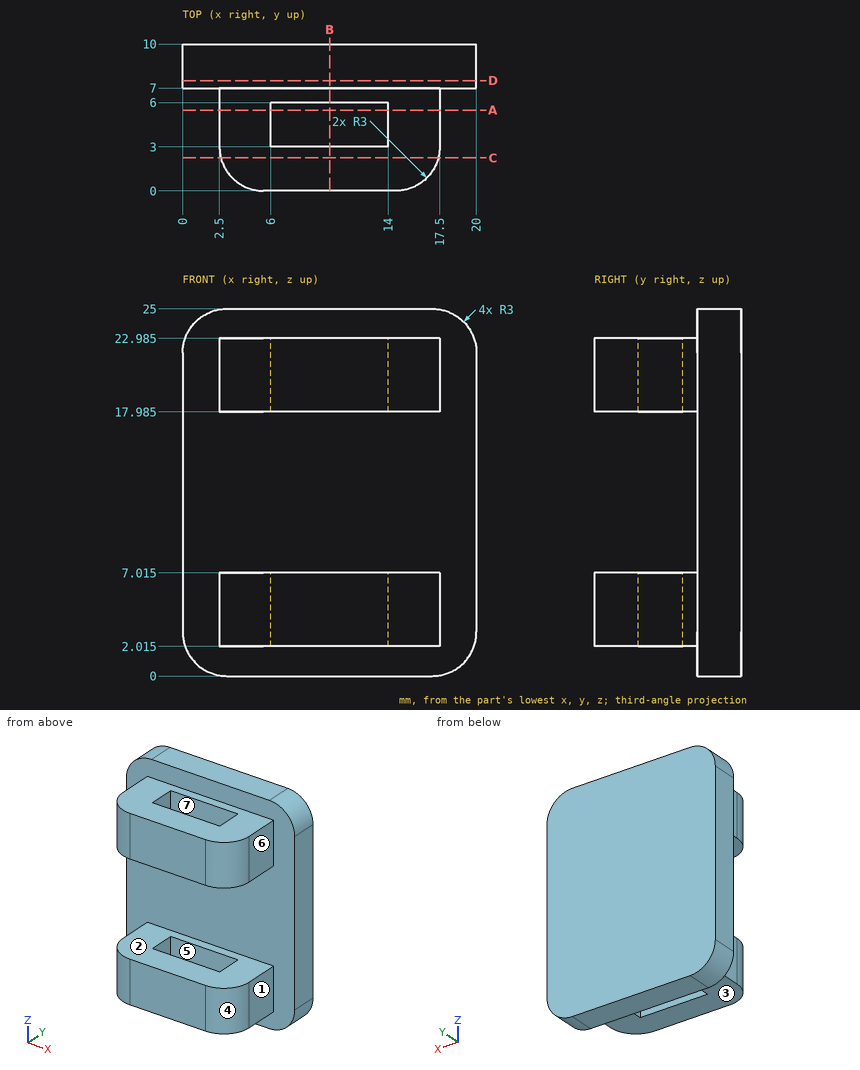
Part print with two shaded views. Sizes in mm from the minimum x, y, z corner. A direction names the side the tool comes from. Give positions to 0.01 mm unless a question says otherwise; leave off trailing zeros. Order: outer loops, then holes, each group sorted by start corner. A loop starts at its lowest first (then second) coordinate and runs counter-clockwise, first axis right, second up. Notation, with made-up numbers: M 67,76 L 125,76 A7 ccw 125,82 Z; hole C 39,3.25 d2. An arc over 180 degrees is marked long. Write item = value, one per line.
Q1. Cut at B-B, the plane x = 10. List the corners of the cut face in (y, z) (3 decimals).
Derived:
outline = M 0,2.015 L 3,2.015 L 3,7.015 L 0,7.015 Z; M 0,17.985 L 3,17.985 L 3,22.985 L 0,22.985 Z; M 6,2.015 L 7,2.015 L 7,0 L 10,0 L 10,25 L 7,25 L 7,22.985 L 6,22.985 L 6,17.985 L 7,17.985 L 7,7.015 L 6,7.015 Z
Q2. Drill centre lines: line 1 (Y direction, x = 11.25, z = 6); line 2 (Z direction, x = 16, y = 3) (3 decimals); line 3 (X direction, y = 5, z = 6). Where is each one in solid material? Low to high. Write a range as [from, to].
Derived:
line_1 = [0, 3], [6, 10]
line_2 = [2.015, 7.015], [17.985, 22.985]
line_3 = [2.5, 6], [14, 17.5]
Q3. Cut at C-C, the plane y = 2.25. List the corners of the cut face in (x, z) (3 decimals), then the cut area to 3 significant figures.
Derived:
outline = M 2.595,2.015 L 17.405,2.015 L 17.405,7.015 L 2.595,7.015 Z; M 2.595,17.985 L 17.405,17.985 L 17.405,22.985 L 2.595,22.985 Z
area = 148 mm2
Q4. Flat gauge pins, fed straight in: pin 1 (3.5 mm diameter, centred on x = 7.5, y = 2, fed in from +Z) (3 decimals); pin 2 (4.5 mm diameter, centred on y = 4.5, z = 5, fed in from -X); pin 3 (1.2 mm diameter, centred on y = 5, z = 20.5, fed in from +X). Where does each tip first touch, or does it go through?
Derived:
pin_1 = 22.985
pin_2 = 2.5
pin_3 = 17.5
Q5. Tool access for the marked faces 1, 2 and 3: list every direction of +Z, -Z, +X, -X, +Y, -Y with a clear straight run to the whole face (end or side of a thin tool).
Derived:
face_1 = +Z, -Z, +X, -Y
face_2 = +X, -X, -Y
face_3 = -Z, +X, -X, -Y
Q6. Cut at A-A, the plane y = 5.5. List the corners of the cut face in (x, z) (3 decimals).
Derived:
outline = M 2.5,2.015 L 6,2.015 L 6,7.015 L 2.5,7.015 Z; M 2.5,17.985 L 6,17.985 L 6,22.985 L 2.5,22.985 Z; M 14,2.015 L 17.5,2.015 L 17.5,7.015 L 14,7.015 Z; M 14,17.985 L 17.5,17.985 L 17.5,22.985 L 14,22.985 Z
Q7. Cut at D-D, the plane y = 7.5. List the corners of the cut face in (x, z).
Derived:
outline = M 0,3 A3 ccw 3,0 L 17,0 A3 ccw 20,3 L 20,22 A3 ccw 17,25 L 3,25 A3 ccw 0,22 Z
Q8. Two-plate mould, pull along Y, no slides. Class the marked faces 4, 5, 6 and 7: pulls with the +Y half, pulls with the -Y half, needs draft (parallel to the pull), parting line crosses it, or undercut.
Derived:
face_4 = pulls with the -Y half
face_5 = undercut
face_6 = needs draft
face_7 = undercut
